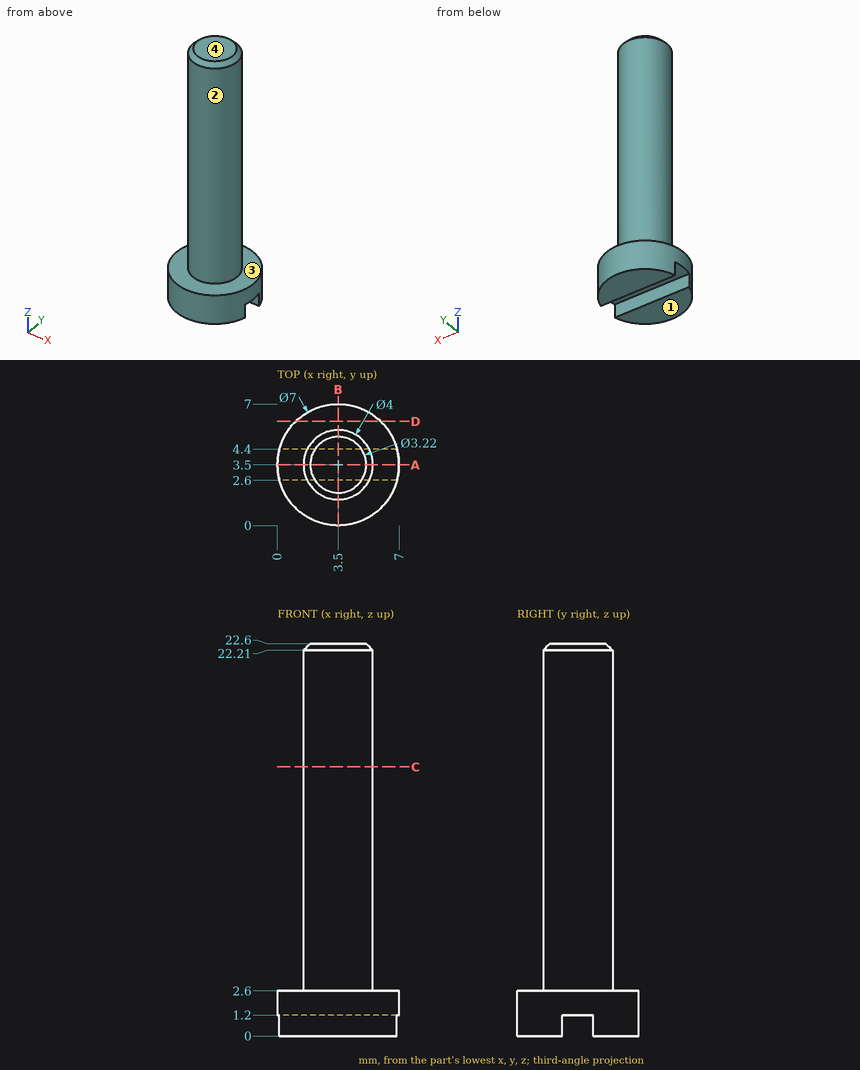
Study the drawing (mm; zero at the part's minimum x, y, z) and answer. A direction names the side the tool comes from. Round coordinates to 2 decimals unless told otherwise and drop trailing zeros. Write each loop counter-clockwise with the first axis right and the second up, starting at its lowest first coordinate (ties: lowest second). Pieces come first, ordered by that corner, then holes.
Q1. Find section A-A on y = 3.5. Determine the outline of the cut face in (x, z).
Values:
outline: (0, 1.2) - (7, 1.2) - (7, 2.6) - (5.5, 2.6) - (5.5, 22.21) - (5.11, 22.6) - (1.89, 22.6) - (1.5, 22.21) - (1.5, 2.6) - (0, 2.6) - close
Q2. Straight lines are drawn through the part: line 1 (Z direction, x = 6.5, y = 3); line 2 (Z direction, x = 5.5, y = 1.5); line 3 (X direction, y = 2.5, z = 13.5). For each, find the intervals that lie inside material, in ascending order.
Values:
line 1: z = 1.2 to 2.6
line 2: z = 0 to 2.6
line 3: x = 1.77 to 5.23
Q3. Find section C-C on z = 15.5. Determine the outline of the cut face in (x, y), and give its area (3 significant figures).
Values:
outline: circle Ø4 at (3.5, 3.5)
area: 12.6 mm2
Q4. The mould has two halves that part along Y. Classify the marked faces 1 and 2: released by +Y, released by -Y, zero draft, split by the parting line, or undercut.
Values:
face 1: zero draft
face 2: split by the parting line
Q5. Find section B-B on x = 3.5. Determine the outline of the cut face in (y, z).
Values:
outline: (0, 0) - (2.6, 0) - (2.6, 1.2) - (4.4, 1.2) - (4.4, 0) - (7, 0) - (7, 2.6) - (5.5, 2.6) - (5.5, 22.21) - (5.11, 22.6) - (1.89, 22.6) - (1.5, 22.21) - (1.5, 2.6) - (0, 2.6) - close
Q6. Flat-ended cylindrical pins translate along their axes: P1, Ø0.5, axis at x = 5, y = 3.5, coming from the -Z side; P2, Ø4, axis at x = 1, z = 3, coming from the +Y side; P3, Ø4, axis at x = 6, z = 16, coming from the +Y side. Find the tip coordinate at first contact, or state that the pin passes through.
Values:
P1: stops at z = 1.2
P2: stops at y = 6.96
P3: stops at y = 5.44
Q7. A tool of negligible diameter and unlimited length cuts with its end or side. For the marked faces 3 and 4, from which of +Z, -Z, +X, -X, +Y, -Y can it reach the whole face along a straight path? Write none if from no direction.
Values:
face 3: +Z
face 4: +Z, +X, -X, +Y, -Y
Q8. Find section D-D on y = 6. Determine the outline of the cut face in (x, z).
Values:
outline: (1.05, 0) - (5.95, 0) - (5.95, 2.6) - (1.05, 2.6) - close
